from build123d import *

# Parameters (mm, degrees)
EXTRUS_O_FINA1_DEPTH  = 20
ESBO_O3_R             = 2
CORTE_EXTRUS_O1_DEPTH = 10


with BuildPart() as part:
    # Esboço1 → Extrusão-Fina1 (new body)
    with BuildSketch(Plane.XY):
        with BuildLine():
            Line((0, 0), (-20, 0))
            ThreePointArc((-20, 0), (-25.656854249, 2.343145751), (-28, 8))
            Line((-28, 8), (-28, 14))
            ThreePointArc((-28, 14), (-25.656854249, 19.656854249), (-20, 22))
            Line((-20, 22), (-2.961110141, 22))
            ThreePointArc((-2.961110141, 22), (-0.581161614, 22.785059097), (0.864586792, 24.832077496))
            Line((0.864586792, 24.832077496), (1.167922504, 25.825696933))
            Line((1.167922504, 25.825696933), (2.124346737, 25.533716307))
            Line((2.124346737, 25.533716307), (1.821011026, 24.54009687))
            ThreePointArc((1.821011026, 24.54009687), (0.013825518, 21.981323872), (-2.961110141, 21))
            Line((-2.961110141, 21), (-20, 21))
            ThreePointArc((-20, 21), (-24.949747468, 18.949747468), (-27, 14))
            Line((-27, 14), (-27, 8))
            ThreePointArc((-27, 8), (-24.949747468, 3.050252532), (-20, 1))
            Line((-20, 1), (0, 1))
            Line((0, 1), (0, 0))
        make_face()
    extrude(amount=EXTRUS_O_FINA1_DEPTH)

    # Esboço3 → Corte-extrusão1 (cut)
    with BuildSketch(Plane.XZ):
        with Locations((-10, 16.395406789)):
            Circle(ESBO_O3_R)
        with Locations((-10, 4.741554418)):
            Circle(ESBO_O3_R)
    extrude(amount=-CORTE_EXTRUS_O1_DEPTH, mode=Mode.SUBTRACT)


solid = part.part
Work out the finished part from the listing and answer in its coordinate system (mm). A direction names the side the tool comes from. Give positions to 0.01 mm unless a question says otherwise; leave off trailing zeros. Loops run counter-clockwise (first coordinate to the right, second up) from the corner with the lowest first, then second, coordinate; pieces in that order, holes last. Notation, with made-up numbers: (65.5, 9) - (98.5, 9) arc R26 ccw to (98.5, 40) - close; hole circle Ø9 at (16, 35). An arc over 180 degrees is marked (long way). Answer in a Markdown table with one row per item. Add a question column.
Q1. The part is cut by section C-C (z = 14). Determine the outline of the cut face in (x, y).
Q2. The part is cut by section B-B (x = -4.5). Determine the outline of the cut face in (y, z).
Q3. Each of these flat-tipped pins is pushed along its axis until it touches: P1, Ø4, axis at y = 21.5, z = 2.5, coming from the +X side; P2, Ø10, axis at x = -11, z = 9, coming from the +Y side; P3, Ø10, axis at y = 3.5, z = 11, coming from the +X side. Where does it stop, or does it pass through?
Q4. A tool of negligible diameter and unlimited length cuts with its end or side. For faces 1 (the flat face through (-10, 0, 10)), 2 (the cylindrical face through (-25, 3.1, 9.9)), 3 (the flat face through (0, 0.5, 9.9)), 4 (the cylindrical face through (-25.594, 2.281, 9.86)), 5 (the flat face through (-12, 22, 10)), from which of +Z, -Z, +X, -X, +Y, -Y can it reach the whole face along a straight path? Write none if from no direction.
Q5. The part is cut by section D-D (x = -23). Determine the outline of the cut face in (y, z).
Q6. The part is cut by section A-A (x = -10). Determine the outline of the cut face in (y, z).
Q7. Determine the mould class of faces 6 (the cylindrical face through (-10.434, 0.493, 14.443)), 7 (the cylindrical face through (-25.719, 19.594, 9.86)), 8 (the flat face through (1.975, 25.044, 9.86)), 9 (the cylindrical face through (-11.587, 0.493, 3.525)) for opening direction X: released by +X, released by -X, zero draft, split by the parting line, or undercut.
Q8. Consider line 1 along Z through (x, y) = (-10, 0.5); line 2 along Y through (x, z) = (-9.5, 10.75); line 3 along Y through (x, z) = (-22.5, 17). Determine where each line is inside the solid, lowest interval first.
Solution:
| question | item | result |
|---|---|---|
| 1 | outline | (-28, 8) arc R8 ccw to (-20, 0) - (0, 0) - (0, 1) - (-20, 1) arc R7 cw to (-27, 8) - (-27, 14) arc R7 cw to (-20, 21) - (-2.96, 21) arc R5 ccw to (1.82, 24.54) - (2.12, 25.53) - (1.17, 25.83) - (0.86, 24.83) arc R4 cw to (-2.96, 22) - (-20, 22) arc R8 ccw to (-28, 14) - close |
| 2 | outline | (0, 0) - (1, 0) - (1, 20) - (0, 20) - close; (21, 0) - (22, 0) - (22, 20) - (21, 20) - close |
| 3 | P1 | stops at x = 1.37 |
| 3 | P2 | stops at y = 22 |
| 3 | P3 | stops at x = 0 |
| 4 | face 1 | +Z, -Z, +X, -X, -Y |
| 4 | face 2 | +Z, -Z, +X |
| 4 | face 3 | +Z, -Z, +X, -Y |
| 4 | face 4 | +Z, -Z, -X, -Y |
| 4 | face 5 | +Z, -Z, -X, +Y |
| 5 | outline | (0.58, 0) - (1.68, 0) - (1.68, 20) - (0.58, 20) - close; (20.32, 0) - (21.42, 0) - (21.42, 20) - (20.32, 20) - close |
| 6 | outline | (0, 0) - (1, 0) - (1, 2.74) - (0, 2.74) - close; (0, 6.74) - (1, 6.74) - (1, 14.4) - (0, 14.4) - close; (0, 18.4) - (1, 18.4) - (1, 20) - (0, 20) - close; (21, 0) - (22, 0) - (22, 20) - (21, 20) - close |
| 7 | face 6 | undercut |
| 7 | face 7 | released by -X |
| 7 | face 8 | released by +X |
| 7 | face 9 | undercut |
| 8 | line 1 | z = 0 to 2.74, 6.74 to 14.4, 18.4 to 20 |
| 8 | line 2 | y = 0 to 1, 21 to 22 |
| 8 | line 3 | y = 0.4 to 1.46, 20.54 to 21.6 |
